Autodesk Inventor part; units mm, degrees
ref_plane "YZ Plane" through (0, 0, 0) normal (1, 0, 0) x (0, 1, 0)
ref_plane "XZ Plane" through (0, 0, 0) normal (0, 1, 0) x (-1, 0, 0)
ref_plane "XY Plane" through (0, 0, 0) normal (0, 0, 1) x (1, 0, 0)
sketch "スケッチ1" plane through (0, 0, 0) normal (1, 0, 0) x (0, 1, 0)
  line L0 (6.1647, 10.3826) -> (-1.9353, 10.3826)
  line L1 (-1.9353, 10.3826) -> (-1.9353, 2.8826)
  line L2 (-1.9353, 2.8826) -> (6.1647, 2.8826)
  line L3 (6.1647, 2.8826) -> (6.1647, 10.3826)
  arc A0 (6.1647, 10.3826) -> (-1.9353, 10.3826) centre (2.1147, 10.3826) ccw
  circle A1 centre (2.1147, 10.3826) radius 1.64
  point P0 (0, 0)
  dimension "d0" = 8.1
  dimension "d1" = 7.5
  dimension "d2" = 3.28
extrude "押し出し1" add sketch "スケッチ1" along normal blind 1.3
sketch "スケッチ2" plane through (1.3, 0, 0) normal (1, 0, 0) x (0, 0, -1)
  point P0 (0, 0)
sketch "スケッチ3" plane through (1.3, 0, 0) normal (1, 0, 0) x (0, 0, -1)
  arc A0 (-10.3826, 6.1647) -> (-10.3826, -1.9353) centre (-10.3826, 2.1147) ccw
  circle A1 centre (-10.3826, 2.1147) radius 1.64
  point P0 (0, 0)
  dimension "d6" = 3.28
hole "穴1" at (1.3, 2.1147, 10.3826) direction (-1, 0, 0) diameter 3.28 depth 1.3
equation "\"BendRadius\" = Thickness"
equation "\"BendReliefWidth\" = Thickness"
equation "\"BendReliefDepth\" = 0.5 * Thickness"
equation "\"CornerReliefSize\" = 4 * Thickness"
equation "\"MinimumRemnant\" = 2 * Thickness"
equation "\"TransitionRadius\" = BendRadius"
equation "\"JacobiRadiusSize\" = BendRadius"
equation "\"GapSize\" = Thickness"
Work out the finished part from the listing and answer in its coordinate system (mm). Give positions to 0.01 mm unless a question says otherwise; leave off trailing zeros. Loops run counter-clockwise (first coordinate to the right, second up) from the corner with the lowest first, then second, coordinate; pieces in that order, holes last. Notation, with made-up numbers: (89, 66) - (145, 66) arc R21 ccw to (145, 88) - close; hole circle Ø7 at (70.25, -9.5). An arc over 180 degrees is marked (long way). Answer in a Markdown table with one row per item. Add a question column.
Q1. The part is cut by section B-B (z = 11.5). Determine the outline of the cut face in (x, y), and give its area (3 significant figures).
Q2. Determine the mould class of faces 1 (the cylindrical face through (0.64, 2.04, 12.02)), 2 (the cylindrical face through (0.64, 2.03, 14.43)), 3 (the flat face through (1, -1.935, 7)) for opening direction Z: released by +Z, released by -Z, zero draft, split by the parting line, or undercut.
Q3. The part is cut by section C-C (x = 0.2). Determine the outline of the cut face in (y, z).
Q4. This flat-tipped pin is pushed along its axis until it touches: P1, Ø2, axis at y = 2.11, z = 10.38, coming from the +X side. Where does it stop, or does it pass through?
Q5. The part is cut by section D-D (y = -0.5). Determine the outline of the cut face in (x, z).
Q6. The part is cut by section A-A (y = 3). Determine the outline of the cut face in (x, z), and give its area (3 significant figures).
Q7. Consider line 1 along Z through (x, y) = (0.25, 1); line 2 along Y through (x, z) = (0.95, 9.5); line 3 along Z through (x, y) = (0.9, 2). Determine where each line is inside the solid, lowest interval first.
Solution:
| question | item | result |
|---|---|---|
| 1 | outline | (0, -1.78) - (1.3, -1.78) - (1.3, 0.91) - (0, 0.91) - close; (0, 3.32) - (1.3, 3.32) - (1.3, 6.01) - (0, 6.01) - close |
| 1 | area | 7.00 mm² |
| 2 | face 1 | undercut |
| 2 | face 2 | released by +Z |
| 2 | face 3 | zero draft |
| 3 | outline | (-1.94, 2.88) - (6.16, 2.88) - (6.16, 10.38) arc R4.05 ccw to (-1.94, 10.38) - close; hole circle Ø3.28 at (2.11, 10.38) |
| 4 | P1 | passes through |
| 5 | outline | (0, 2.88) - (1.3, 2.88) - (1.3, 13.48) - (0, 13.48) - close |
| 6 | outline | (0, 2.88) - (1.3, 2.88) - (1.3, 9) - (0, 9) - close; (0, 11.76) - (1.3, 11.76) - (1.3, 14.33) - (0, 14.33) - close |
| 6 | area | 11.3 mm² |
| 7 | line 1 | z = 2.88 to 9.18, 11.59 to 14.28 |
| 7 | line 2 | y = -1.94 to 0.73, 3.5 to 6.16 |
| 7 | line 3 | z = 2.88 to 8.75, 12.02 to 14.43 |
